Can you work these out from the model? Positions are in its coordinate system, mm. A direction names the side the tool comes from. Round coordinates to 2 decimals unless told otherwise and drop trailing zeros. Order: outer loops, then holes, each group sorted by start corner. A loop starts at its lowest first (then second) coordinate and runs counter-clockwise, first axis right, second up. Notation, with made-up numbers: (48.5, 4) -> (83.5, 4) arc R23 ccw to (83.5, 14) -> close; hole circle Ø9 at (10.5, 4). An arc over 180 degrees is marked (long way). Use a Markdown table: item, result. Add a question column.
Q1. I'm going to push flat-ended pins straight in: pin 1 Ø6.5 at (y, z) = (8, 7.5) entering from -X; pin 2 Ø2 at (x, y) = (9.5, 6.5) entering from -Z; pin 3 Ø1 at (x, z) = (6.5, 9) entering from +Y; pin 4 Ø3 at (x, z) = (8, 4) entering from +Y. Where does each tip first touch, or does it pass through?
Q2. If we section it at B-B on y = 1.5: List the corners of the cut face in (x, z) for me.
Q3. We'd pull the mould along X, two halves only. Please class faces 3 (the face through (5, 4, 6)), 4 (the face through (8.5, 4, 9)), 5 (the face through (11, 15, 7.5)), 6 (the face through (0, 3, 7)): +X half, -X half, draft (parallel to the pull), parting line (faces both ways), or undercut.
Q4. If we section it at C-C on x = 4.25: List the corners of the cut face in (y, z) for me.
Q5. If we section it at D-D on y = 10.5: List the corners of the cut face in (x, z) for me, plus the area to 3 significant figures.
Q6. For faces 1 (the face through (7, 0, 7)), 2 (the face through (7, -1, 15)), which set-ups out of +Z, -Z, +X, -X, +Y, -Y let a thin tool reach every point of the face, with its end or its side?
Q7. If we section it at A-A on z = 7.5: List the corners of the cut face in (x, y) for me.
Q8. I need wall thicknesses on line 1 along Y through (x, z) = (10.95, 7.5); line 2 along X through (y, z) = (0.75, 4); line 3 along Z through (x, y) = (10.1, 8). Which ranges of each line are inside material? Lowest first, please. Write a range as [from, to].
Solid Edge part; units mm, degrees
sketch "Sketch1" plane through (0, 0, 0) normal (0, -1, 0) x (1, 0, 0)
  line L0 (13.5, 0) -> (0, 0)
  line L1 (0, 0) -> (0, 15)
  line L2 (0, 15) -> (13.5, 15)
  line L3 (13.5, 15) -> (13.5, 0)
extrude "Protrusion1" add sketch "Sketch1" along normal blind 5
sketch "Sketch2" plane through (18.75, 0, 7.5) normal (0, 1, 0) x (-1, 0, 0)
  line L0 (13.75, -7.5) -> (13.75, 7.5)
  line L1 (13.75, 7.5) -> (18.75, 7.5)
  line L2 (18.75, 7.5) -> (18.75, -7.5)
  line L3 (18.75, -7.5) -> (13.75, -7.5)
extrude "ExtrudedProtrusion_3" add sketch "Sketch2" along normal blind 15
sketch "Sketch3" plane through (0, 5, 7.5) normal (-1, 0, 0) x (0, -1, 0)
  circle A0 centre (-3, 0) radius 4
extrude "Cutout1" cut sketch "Sketch3" against normal through all
fillet "Round1" radius 7 2 edges at (2.5, 15, 15) (2.5, 15, 0)
mirror "Mirror1" about plane through (6.75, 5, 7.5) normal (-1, 0, 0) of "ExtrudedProtrusion_3", "Cutout1"
fillet "Round2" radius 7 2 edges at (11, 15, 15) (11, 15, 0)
Answer below:
| question | item | result |
|---|---|---|
| 1 | pin 1 | through |
| 1 | pin 2 | z = 0 |
| 1 | pin 3 | y = 0 |
| 1 | pin 4 | y = 14.82 |
| 2 | outline | (0, 0) -> (5, 0) -> (5, 15) -> (0, 15) -> close; (8.5, 0) -> (13.5, 0) -> (13.5, 15) -> (8.5, 15) -> close |
| 3 | face 3 | undercut |
| 3 | face 4 | undercut |
| 3 | face 5 | draft |
| 3 | face 6 | -X half |
| 4 | outline | (-5, 0) -> (8, 0) arc R7 ccw to (15, 7) -> (15, 8) arc R7 ccw to (8, 15) -> (-5, 15) -> close; hole circle Ø8 at (8, 7.5) |
| 5 | outline | (0, 0.46) -> (5, 0.46) -> (5, 4.38) -> (0, 4.38) -> close; (0, 10.62) -> (5, 10.62) -> (5, 14.54) -> (0, 14.54) -> close; (8.5, 0.46) -> (13.5, 0.46) -> (13.5, 4.38) -> (8.5, 4.38) -> close; (8.5, 10.62) -> (13.5, 10.62) -> (13.5, 14.54) -> (8.5, 14.54) -> close |
| 5 | area | 78.3 mm² |
| 6 | face 1 | +Z, -Z, +Y |
| 6 | face 2 | +Z, +X, -X, +Y, -Y |
| 7 | outline | (0, -5) -> (13.5, -5) -> (13.5, 4) -> (8.5, 4) -> (8.5, 0) -> (5, 0) -> (5, 4) -> (0, 4) -> close; (0, 12) -> (5, 12) -> (5, 15) -> (0, 15) -> close; (8.5, 12) -> (13.5, 12) -> (13.5, 15) -> (8.5, 15) -> close |
| 8 | line 1 | [-5, 4], [12, 15] |
| 8 | line 2 | [0, 5], [8.5, 13.5] |
| 8 | line 3 | [0, 3.5], [11.5, 15] |
